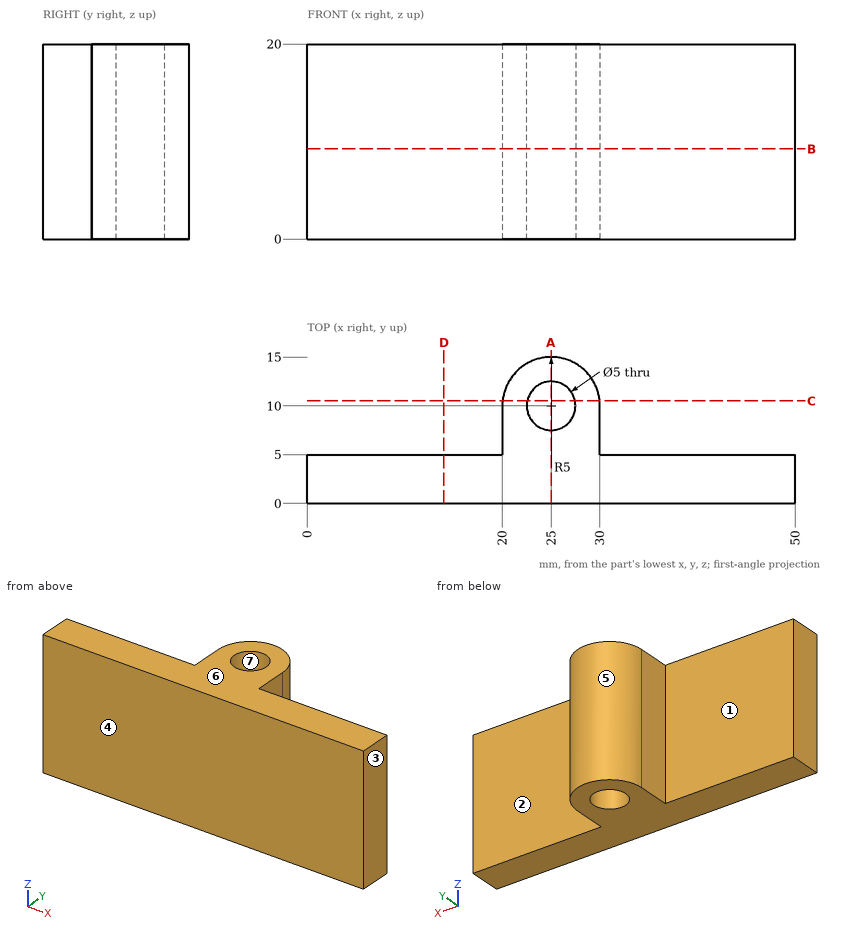
Design review of the part shown in the three views and the two pictorial views. Dimensions are in mm from the part's minimum x, y and z. A direction names the side the tool comes from. Give positions to 0.01 mm unless a question says otherwise; leave off trailing zeros. Loops run counter-clockwise (first coordinate to the right, second up) from the corner with the lowest first, then second, coordinate; pieces in that order, holes last. Notation, with made-up numbers: M 68,-35 L 108,-35 A7 ccw 108,-25 Z; hole C 56.5,11 d8. An arc over 180 degrees is marked long. Put each result on its own line as item: value. Start each with the question number.
(1) Add section B-B, the plane z = 9.25. Write out the cut boundary in (x, y).
(2) Add section A-A, the plane x = 25. Write out the cut boundary in (y, z), then the cut area to 3 significant figures.
(3) Wall thickness on L1, parallel to Y at x = 25, z = 11.5; L2, parallel to Y at x = 17.5, z = 18.25; L3, parallel to X at y = 5.25, z = 7.5: over which ranges is each line inside the solid? List them lowest first.
(4) Add section C-C, the plane y = 10.5. Write out the cut boundary in (x, z), then the cut area to 3 significant figures.
(5) Machinability: for the marked faces 1, 2 and 3, which of the approach directions +Z, -Z, +X, -X, +Y, -Y give a long, thin tool a straight path to every point of the face, cutting with its end or side? Answer none if there is none.
(6) Add section D-D, the plane x = 14. Write out the cut boundary in (y, z).
(7) For pin 1 (2.5 mm diameter, centred on y = 8.5, z = 8, fed in from -X); pin 2 (2 mm diameter, centred on x = 41.5, z = 12.5, fed in from +Y); pin 3 (3 mm diameter, centred on y = 10, z = 14, fed in from +X), all flat-tipped, find the tip position at first contact; note any pin that passes through.
(8) The part is to be moulded in two halves that separate along Y. For the marked faces 4, 5, 6 and 7, say which applies: +Y half, -Y half, draft (parallel to the pull), parting line (faces both ways), or undercut.
Result:
1. outline: M 0,0 L 50,0 L 50,5 L 30,5 L 30,10 A5 ccw 20,10 L 20,5 L 0,5 Z; hole C 25,10 d5
2. outline: M 0,0 L 7.5,0 L 7.5,20 L 0,20 Z; M 12.5,0 L 15,0 L 15,20 L 12.5,20 Z
2. area: 200 mm^2
3. L1: y = 0 to 7.5, 12.5 to 15
3. L2: y = 0 to 5
3. L3: x = 20 to 30
4. outline: M 20.03,0 L 22.55,0 L 22.55,20 L 20.03,20 Z; M 27.45,0 L 29.97,0 L 29.97,20 L 27.45,20 Z
4. area: 101 mm^2
5. face 1: +Z, -Z, -X, +Y
5. face 2: +Z, -Z, +X, +Y
5. face 3: +Z, -Z, +X, +Y, -Y
6. outline: M 0,0 L 5,0 L 5,20 L 0,20 Z
7. pin 1: stops at x = 20
7. pin 2: stops at y = 5
7. pin 3: stops at x = 30
8. face 4: -Y half
8. face 5: +Y half
8. face 6: draft
8. face 7: undercut
